Could you check a few things on this model? Use its own coordinates, in mm. A direction names the side the tool comes from. Coordinates: 2 decimals unless noted, no trailing zeros. Loops run counter-clockwise (first coordinate to the right, second up) from the corner with the lowest first, then second, coordinate; pieces in that order, holes last. Notation, with made-up numbers: M 32,4 L 59,4 A32 ccw 59,34 Z; hole C 52.5,84 d10. An arc over 180 degrees is marked long. Return JSON: item names as keys, results as strings. Group by question number.
from build123d import *

# Parameters (mm, degrees)
F0_R     = 184.15
F0_R_2   = 76.2
F1_DEPTH = 88.9
F2_R     = 76.2
F3_DEPTH = 76.2
F4_R     = 12.7
F5_DEPTH = 76.2
F6_R     = 12.7
F7_DEPTH = 76.2


with BuildPart() as f1:
    # F0 (on Front) → F1 (new body, symmetric)
    with BuildSketch(Plane.XZ):
        Circle(F0_R)
        Circle(F0_R_2, mode=Mode.SUBTRACT)
    extrude(amount=F1_DEPTH, both=True)

    # F2 (on Front) → F3 (join, symmetric)
    with BuildSketch(Plane.XZ):
        Circle(F2_R)
    extrude(amount=F3_DEPTH, both=True)

    # F4 (on face) → F5 (cut, symmetric)
    with BuildSketch(Plane.XZ.offset(76.2)):
        Circle(F4_R)
    extrude(amount=F5_DEPTH, both=True, mode=Mode.SUBTRACT)

    # F6 (on face) → F7 (cut, symmetric)
    with BuildSketch(Plane.XZ):
        Circle(F6_R)
    extrude(amount=F7_DEPTH, both=True, mode=Mode.SUBTRACT)


solid = f1.part
(1) Imagine slicing it at A-A, the plane z = 0. Write out the boundary of the cut face in (x, y).
(2) We'd pull the mould along Z, two halves only. Please class faces 1 (the face through (-146.1, -1.2, -112.1)), 2 (the face through (-2.75, -1.07, -12.4)), 3 (the face through (79, -88.9, 3)): +Z half, -Z half, draft (parallel to the pull), parting line (faces both ways), or undercut.
(3) Imagine slicing it at B-B, the plane x = 0. Write out the boundary of the cut face in (y, z), then the cut area to 3 significant figures.
(4) Imagine slicing it at D-D, the plane z = -55. Write out the boundary of the cut face in (x, y).
(5) For faces 4 (the face through (79, 88.9, 3)), 5 (the face through (16, 76.2, 1)), 6 (the face through (-60.47, -82.461, -46.367)), which set-ups out of +Z, -Z, +X, -X, +Y, -Y let a thin tool reach every point of the face, with its end or its side?
(6) Imagine slicing it at C-C, the plane y = 35.5. Write out the boundary of the cut face in (x, z), then the cut area to 3 significant figures.
(7) Will these pins go through, and if not, where does the flat tip stop? P1, Ø5, axis at y = -24.5, z = 113.5, coming from the +X side; P2, Ø3, axis at y = 16, z = 23, coming from the +X side; P3, Ø1, axis at y = -45, z = 145.5, coming from the -X side; P4, Ø15, axis at x = 0, z = 0, coming from the +Y side.
(8) If I drill on L1, parallel to Z at x = 0, y = 81; L2, parallel to Z at x = 0, y = 27; L3, parallel to Y at x = 31.5, z = -24.5, over which ranges is the centre line in solid material (lowest first)? Write a range as [from, to].
Checks:
{
 "1": {"outline": "M -184.15,-88.9 L -76.2,-88.9 L -76.2,-76.2 L -12.7,-76.2 L -12.7,76.2 L -76.2,76.2 L -76.2,88.9 L -184.15,88.9 Z; M 12.7,-76.2 L 76.2,-76.2 L 76.2,-88.9 L 184.15,-88.9 L 184.15,88.9 L 76.2,88.9 L 76.2,76.2 L 12.7,76.2 Z"},
 "2": {"face 1": "parting line", "face 2": "undercut", "face 3": "draft"},
 "3": {"outline": "M -88.9,-184.15 L 88.9,-184.15 L 88.9,-76.2 L 76.2,-76.2 L 76.2,-12.7 L -76.2,-12.7 L -76.2,-76.2 L -88.9,-76.2 Z; M -88.9,76.2 L -76.2,76.2 L -76.2,12.7 L 76.2,12.7 L 76.2,76.2 L 88.9,76.2 L 88.9,184.15 L -88.9,184.15 Z", "area": "57,700 mm²"},
 "4": {"outline": "M -175.74,-88.9 L -52.74,-88.9 L -52.74,-76.2 L 52.74,-76.2 L 52.74,-88.9 L 175.74,-88.9 L 175.74,88.9 L 52.74,88.9 L 52.74,76.2 L -52.74,76.2 L -52.74,88.9 L -175.74,88.9 Z"},
 "5": {"face 4": "+Z, -Z, +X, -X, +Y", "face 5": "+Y", "face 6": "-Y"},
 "6": {"outline": "C 0,0 d368.3; hole C 0,0 d25.4", "area": "106,000 mm²"},
 "7": {"P1": "x = 146.94", "P2": "x = 182.89", "P3": "x = -113.52", "P4": "through"},
 "8": {"L1": "[-184.15, -76.2], [76.2, 184.15]", "L2": "[-184.15, -12.7], [12.7, 184.15]", "L3": "[-76.2, 76.2]"}
}
